The drawing under review shows one solid part. Ordinate dimensions are in mm from its lowest x, y, z. Round coordinates to 2 decimals unless told otherwise and drop trailing zeros. Write each loop counter-clockwise with the first axis right and the second up, starting at its lowest first coordinate (ties: lowest second). Pieces come first, ordered by that corner, then holes. Notation, with made-up numbers: (71.5, 83.25) -> (75.5, 83.25) arc R30 ccw to (75.5, 106.25) -> close; hole circle Ø3 at (-26.5, 29.5). An arc over 180 degrees is marked (long way). Answer in a Markdown table with one row per item.
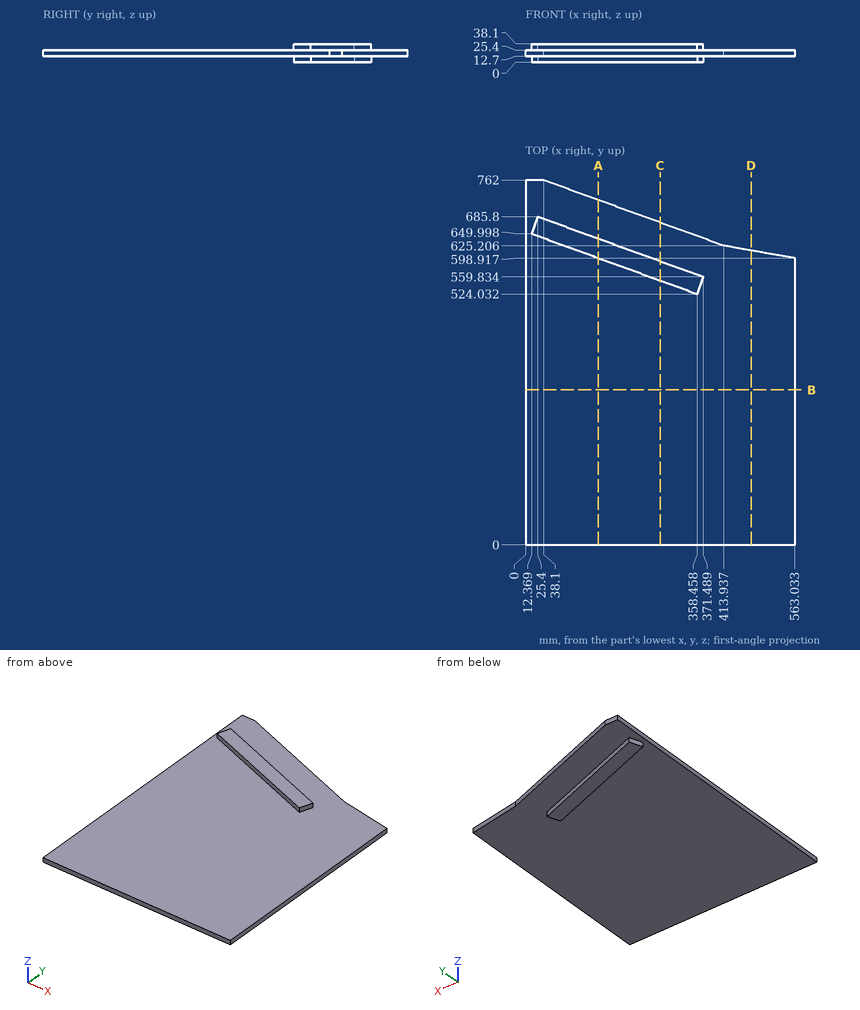
1) Clearance check with flat-ended pins moving along their axes: pin 1 Ø3 at (x, y) = (166.5, 234.5) entering from -Z; pin 2 Ø8 at (x, z) = (317.5, 9) entering from +Y; pin 3 Ø1.5 at (x, y) = (294.5, 376.5) entering from +Z. State where each tip first meets the part, or that it passes through.
Solved:
| item | result |
|---|---|
| pin 1 | z = 12.7 |
| pin 2 | y = 660.86 |
| pin 3 | z = 25.4 |
2) Consider section C-C on x = 281. State the section outline as (y, z) points.
Solved:
| item | result |
|---|---|
| outline | (0, 12.7) -> (552.22, 12.7) -> (552.22, 0) -> (592.77, 0) -> (592.77, 12.7) -> (673.59, 12.7) -> (673.59, 25.4) -> (592.77, 25.4) -> (592.77, 38.1) -> (552.22, 38.1) -> (552.22, 25.4) -> (0, 25.4) -> close |
3) Consider section D-D on x = 471.5. State the section outline as (y, z) points, then the cut area to 3 significant figures.
Solved:
| item | result |
|---|---|
| outline | (0, 12.7) -> (615.06, 12.7) -> (615.06, 25.4) -> (0, 25.4) -> close |
| area | 7,810 mm² |
4) For line 1 (Z direction, x = 411, y = 625); line 2 (Y direction, x = 99.5, z = 24.5); line 3 (Y direction, x = 365, z = 22), list the stretches that pass through material, from the lowest coordinate up. Write a range as [from, to].
Solved:
| item | result |
|---|---|
| line 1 | [12.7, 25.4] |
| line 2 | [0, 739.65] |
| line 3 | [0, 643.02] |
5) Consider section A-A on x = 152. State the section outline as (y, z) points, then the cut area to 3 significant figures.
Solved:
| item | result |
|---|---|
| outline | (0, 12.7) -> (599.18, 12.7) -> (599.18, 0) -> (639.72, 0) -> (639.72, 12.7) -> (720.54, 12.7) -> (720.54, 25.4) -> (639.72, 25.4) -> (639.72, 38.1) -> (599.18, 38.1) -> (599.18, 25.4) -> (0, 25.4) -> close |
| area | 10,200 mm² |
6) Consider section B-B on y = 324. State the section outline as (x, z) points.
Solved:
| item | result |
|---|---|
| outline | (0, 12.7) -> (563.03, 12.7) -> (563.03, 25.4) -> (0, 25.4) -> close |
